Verification items for the finished model (mm, model axes). A direction names the side the tool comes from. Round coordinates to 2 decimals unless told otherwise and drop trailing zeros. Write each loop counter-clockwise with the first axis right and the second up, starting at its lowest first coordinate (ties: lowest second). Pieces come first, ordered by that corner, then holes. Notation, with made-up numbers: (77.25, -4.5) -> (94.25, -4.5) arc R24 cw to (94.25, 30.5) -> close; hole circle Ø3 at (77, 21.25). An arc over 180 degrees is marked (long way). Answer as a JSON object with one key per item and string values. Group by question number.
(1) Draft check along Y on faces 6 (the face through (19.4, 0.3, 4.6)), 7 (the face through (27.626, 3.102, 1.726)), 8 (the face through (-6.39, -2.86, 0.99)). Enter one of: released by +Y, released by -Y, zero draft, split by the parting line, or undercut.
(2) Sectioned sample at A-A on z = 2.75. Record the cut outline in (x, y).
(3) Sectioned sample at D-D on x = -0.5. Record the cut outline in (y, z), and give its area (3 significant figures).
(4) Scan lines: L1, parallel to Y at x = 0, z = 1.2; L2, parallel to Y at x = 12, z = 4.2; L3, parallel to Y at x = 27, z = 3.75. Record each from-to range of solid material in increasing order. Write a range as from..to.
(5) Set-up check for faces 1 (the face through (1, 0, 2)), 2 (the face through (29.343, 7, 3)), 3 (the face through (31.6, 0.1, 3.5)), 4 (the face through (6, 5.127, 4)), 5 (the face through (9.98, 7.94, 6.25)): record each of +Z, -Z, +X, -X, +Y, -Y from which the full face is reachable in a straight line by a thin tool's end or side.
(6) Gauge pin test, flat ends, axial feed: pin 1 Ø1.8 at (y, z) = (-5, 2.5) entering from +X; pin 2 Ø5.5 at (x, y) = (32, 1.5) entering from -Z; pin 3 Ø1.5 at (x, y) = (18, -1) entering from -Z. Record the tip position at first contact, or that the pin passes through.
```python
from build123d import *

# Parameters (mm, degrees)
BOSS_EXTRUDE1_DEPTH = 2
BOSS_EXTRUDE2_DEPTH = 1.5
BOSS_EXTRUDE3_DEPTH = 2.3
SKETCH6_W           = 5.48
SKETCH6_H           = 3
CUT_EXTRUDE1_DEPTH  = 3.8
SKETCH7_R           = 3
CUT_EXTRUDE2_DEPTH  = 3.3
SKETCH8_W           = 22.343145751
SKETCH8_H           = 2
SKETCH8_W_2         = 17.500252532
SKETCH8_H_2         = 1.5
BOSS_EXTRUDE4_DEPTH = 1.2
SKETCH9_R           = 2.5
BOSS_EXTRUDE5_DEPTH = 1.2
SKETCH10_R          = 0.95
CUT_EXTRUDE3_DEPTH  = 8.2
SKETCH11_R          = 2
CUT_EXTRUDE4_DEPTH  = 2.2
SKETCH12_R          = 3.9
BOSS_EXTRUDE6_DEPTH = 1.2
CUT_EXTRUDE5_DEPTH  = 3.2
FILLET1_R           = 1.5
FILLET2_R           = 1
SKETCH15_R          = 0.75
CUT_EXTRUDE6_DEPTH  = 10


with BuildPart() as part:
    # Sketch2 → Boss-Extrude1 (new body)
    with BuildSketch(Plane.XY):
        with BuildLine():
            Line((0, 7), (3, 7.456854249))
            Line((3, 7.456854249), (29.343145751, 7.456854249))
            Line((29.343145751, 7.456854249), (29.343145751, 5.656854249))
            ThreePointArc((29.343145751, 5.656854249), (27.60896374, 3.061467459), (27, 0))
            Line((27, 0), (26, -2.543145751))
            Line((26, -2.543145751), (26, -7.043145751))
            Line((26, -7.043145751), (8.499747468, -7.043145751))
            Line((8.499747468, -7.043145751), (4.949747468, -4.949747468))
            ThreePointArc((4.949747468, -4.949747468), (-6.467156728, -2.678784027), (0, 7))
        make_face()
    extrude(amount=BOSS_EXTRUDE1_DEPTH)

    # Sketch3 → Boss-Extrude2 (add)
    with BuildSketch(Plane.XY.offset(2)):
        with BuildLine():
            Line((29.343145751, 7.456854249), (29.343145751, 5.656854249))
            ThreePointArc((29.343145751, 5.656854249), (27.60896374, 3.061467459), (27, 0))
            Line((27, 0), (26, -2.543145751))
            Line((26, -2.543145751), (26, -7.043145751))
            Line((26, -7.043145751), (26, -8.543145751))
            Line((26, -8.543145751), (8.499747468, -8.543145751))
            Line((8.499747468, -8.543145751), (8.499747468, -7.043145751))
            Line((8.499747468, -7.043145751), (6.724747468, -5.996446609))
            Line((6.724747468, -5.996446609), (6.724747468, 2.126854249))
            Line((6.724747468, 2.126854249), (3, 2.126854249))
            Line((3, 2.126854249), (3, 7.456854249))
            Line((3, 7.456854249), (3, 8.956854249))
            Line((3, 8.956854249), (29.343145751, 8.956854249))
            Line((29.343145751, 8.956854249), (29.343145751, 7.456854249))
        make_face()
    extrude(amount=BOSS_EXTRUDE2_DEPTH)

    # Sketch5 → Boss-Extrude3 (add)
    with BuildSketch(Plane.XY.offset(3.5)):
        with BuildLine():
            Line((3, 7.5), (3, 2.126854249))
            Line((3, 2.126854249), (6.724747468, 2.126854249))
            Line((6.724747468, 2.126854249), (6.724747468, -5.996446609))
            Line((6.724747468, -5.996446609), (8.499747468, -7.043145751))
            Line((8.499747468, -7.043145751), (8.499747468, -8.543145751))
            Line((8.499747468, -8.543145751), (26, -8.543145751))
            Line((26, -8.543145751), (26, -5.663145751))
            Line((26, -5.663145751), (35.003145751, -5.663145751))
            ThreePointArc((35.003145751, -5.663145751), (40.663145751, -0.003145751), (35.003145751, 5.656854249))
            Line((35.003145751, 5.656854249), (29.343145751, 5.656854249))
            Line((29.343145751, 5.656854249), (29.343145751, 7.5))
            Line((29.343145751, 7.5), (29.343145751, 8.956854249))
            Line((29.343145751, 8.956854249), (3, 8.956854249))
            Line((3, 8.956854249), (3, 7.5))
        make_face()
    extrude(amount=BOSS_EXTRUDE3_DEPTH)

    # Sketch6 → Cut-Extrude1 (cut)
    with BuildSketch(Plane.XY.offset(5.8)):
        with Locations((5.74, 3.626854249)):
            Rectangle(SKETCH6_W, SKETCH6_H)
    extrude(amount=-CUT_EXTRUDE1_DEPTH, mode=Mode.SUBTRACT)

    # Sketch7 → Cut-Extrude2 (cut)
    with BuildSketch(Plane.XY.offset(5.8)):
        with Locations((35.003145751, -0.003145751)):
            Circle(SKETCH7_R)
    extrude(amount=-CUT_EXTRUDE2_DEPTH, mode=Mode.SUBTRACT)

    # Sketch8 → Boss-Extrude4 (add)
    with BuildSketch(Plane.XY.offset(5.8)):
        with Locations((18.171572876, 7.956854249)):
            Rectangle(SKETCH8_W, SKETCH8_H)
        with Locations((17.249873734, -7.793145751)):
            Rectangle(SKETCH8_W_2, SKETCH8_H_2)
        with BuildLine():
            Line((6.724747468, -4.169704782), (24.343145751, -4.169704782))
            ThreePointArc((24.343145751, -4.169704782), (25.343145751, -3.169704782), (24.343145751, -2.169704782))
            Line((24.343145751, -2.169704782), (6.724747468, -2.169704782))
            Line((6.724747468, -2.169704782), (6.724747468, -4.169704782))
        make_face()
        with BuildLine():
            Line((24.343145751, 4.180295218), (10.48, 4.180295218))
            Line((10.48, 4.180295218), (10.48, 2.180295218))
            Line((10.48, 2.180295218), (24.343145751, 2.180295218))
            ThreePointArc((24.343145751, 2.180295218), (25.343145751, 3.180295218), (24.343145751, 4.180295218))
        make_face()
    extrude(amount=BOSS_EXTRUDE4_DEPTH)

    # Sketch9 → Boss-Extrude5 (add)
    with BuildSketch(Plane.XY.offset(5.8)):
        with Locations((18.5, 0)):
            Circle(SKETCH9_R)
        with Locations((12, 0)):
            Circle(SKETCH9_R)
    extrude(amount=BOSS_EXTRUDE5_DEPTH)

    # Sketch10 → Cut-Extrude3 (cut)
    with BuildSketch(Plane.XY.offset(7)):
        with Locations((18.5, 0)):
            Circle(SKETCH10_R)
        with Locations((12, 0)):
            Circle(SKETCH10_R)
    extrude(amount=-CUT_EXTRUDE3_DEPTH, mode=Mode.SUBTRACT)

    # Sketch11 → Cut-Extrude4 (cut)
    with BuildSketch(Plane(origin=(0, 0, 0), x_dir=(-1, 0, 0), z_dir=(0, 0, -1))):
        with Locations((-12, 0)):
            Circle(SKETCH11_R)
        with Locations((-18.5, 0)):
            Circle(SKETCH11_R)
    extrude(amount=-CUT_EXTRUDE4_DEPTH, mode=Mode.SUBTRACT)

    # Sketch12 → Boss-Extrude6 (add)
    with BuildSketch(Plane.XY.offset(2)):
        Circle(SKETCH12_R)
    extrude(amount=BOSS_EXTRUDE6_DEPTH)

    # Sketch14 → Cut-Extrude5 (cut)
    with BuildSketch(Plane.XY.offset(3.2)):
        with BuildLine():
            Line((1, 0.979795897), (1, -0.979795897))
            ThreePointArc((1, -0.979795897), (-1.4, 0), (1, 0.979795897))
        make_face()
    extrude(amount=-CUT_EXTRUDE5_DEPTH, mode=Mode.SUBTRACT)

    # Fillet1
    fillet1_edges = [part.edges().sort_by_distance(p)[0] for p in [
        (16.171572875, 8.956854249, 2),
        (17.249873734, -8.543145751, 2),
    ]]
    fillet(fillet1_edges, radius=FILLET1_R - 0.0001)  # a hair under: the kernel refuses the full size

    # Fillet2
    fillet2_edges = [part.edges().sort_by_distance(p)[0] for p in [
        (17.249873734, -7.043145751, 0),
        (16.171572875, 7.456854249, 0),
    ]]
    fillet(fillet2_edges, radius=FILLET2_R)

    # Sketch15 → Cut-Extrude6 (cut)
    with BuildSketch(Plane.XZ.offset(-6.956854249)):
        with Locations((10, 7)):
            Circle(SKETCH15_R)
    extrude(amount=-CUT_EXTRUDE6_DEPTH, mode=Mode.SUBTRACT)


solid = part.part
```
Computed values:
{
 "1": {"face 6": "undercut", "face 7": "released by -Y", "face 8": "split by the parting line"},
 "2": {"outline": "circle Ø7.8 at (0, 0); (3, 5.13) -> (8.48, 5.13) -> (8.48, 2.13) -> (6.72, 2.13) -> (6.72, -6) -> (8.5, -7.04) -> (8.5, -8.34) -> (26, -8.34) -> (26, -2.54) -> (27, 0) arc R8 cw to (29.34, 5.66) -> (29.34, 8.76) -> (3, 8.76) -> close; hole (1, -0.98) -> (1, 0.98) arc R1.4 ccw (long way) to start; hole circle Ø1.9 at (12, 0); hole circle Ø1.9 at (18.5, 0)"},
 "3": {"outline": "(-6.98, 0) -> (-1.31, 0) -> (-1.31, 3.2) -> (-3.87, 3.2) -> (-3.87, 2) -> (-6.98, 2) -> close; (1.31, 0) -> (6.46, 0) arc R1 ccw to (6.98, 0.15) -> (6.98, 2) -> (3.87, 2) -> (3.87, 3.2) -> (1.31, 3.2) -> close", "area": "28.8 mm2"},
 "4": {"L1": "-7..-1.4, 1.4..7", "L2": "-8.54..-0.95, 0.95..8.96", "L3": "-5.66..8.96"},
 "5": {"face 1": "+Z, -Z", "face 2": "+Z, -Z, +X, +Y", "face 3": "-Z, +X, -Y", "face 4": "+Z, -X", "face 5": "+Z, +Y"},
 "6": {"pin 1": "x = 26", "pin 2": "z = 3.5", "pin 3": "z = 2.2"}
}
